Geometry: final body of the model. Coordinates: model frame, mm. Round coordinates to 2 decimals unless told otherwise and drop trailing zeros. Order: outer loops, then holes, each group sorted by start corner. A loop starts at its lowest first (then second) coordinate and runs counter-clockwise, first axis right, second up. Notation, with made-up numbers: (73.25, 42.25) - (129.25, 42.25) arc R28 ccw to (129.25, 77.25) - close; hole circle Ø10 at (3, 32). An arc over 180 degrees is marked (long way). Put each result on its own line as item: value. Start each with the question number.
(1) Section A-A (x = -83.5). Output: boundary loops of the cut face in (y, z) (3 decimals).
(2) Material intervals for L1, parallel to X at y = -2.5, z = -4.5; L2, parallel to Z at x = -83, y = -0.8, sorted ascending. Write a range as [from, to].
(3) Pin query (flat end, axial travel): P1, Ø1.5, axis at y = -2, z = -2.5, coming from the -X side; P2, Ø1.6, axis at x = 206.5, y = -1, coming from the -Z side; P3, Ø1, axis at y = -1.5, z = -39.5, coming from the +X side. Return the tip coordinate at first contact, or that it passes through.
from build123d import *

# Parameters (mm, degrees)
F1_DEPTH = 3.175


# Not quite as in the source:
# - ends of sketch curves that miss each other by under 0.0002 mm in the source are joined


with BuildPart() as f1:
    # F0 (on Front) → F1 (new body)
    with BuildSketch(Plane.XZ):
        Polygon((148.5900335276, 41.2750068545), (123.8250335276, 41.2750068545), (123.8250335276, 38.1000068545), (99.0600335276, 38.1000068545), (99.0600335276, 41.2750068545), (74.2950335276, 41.2750068545), (74.2950335276, 38.1000068545), (49.5300335276, 38.1000068545), (49.5300335276, 41.2750068545), (24.7650335276, 41.2750068545), (24.7650335276, 38.1000068545), (3.35276e-05, 38.1000068545), (3.35276e-05, 41.2750068545), (-24.7649664724, 41.2750068545), (-24.7649664724, 38.1000068545), (-49.5299664724, 38.1000068545), (-49.5299664724, 41.2750068545), (-74.2949664724, 41.2750068545), (-74.2949664724, 38.1000068545), (-99.0599664724, 38.1000068545), (-99.0599664724, 41.2750068545), (-123.8249664724, 41.2750068545), (-123.8249664724, 38.1000068545), (-148.5899664724, 38.1000068545), (-148.5899664724, 41.2750068545), (-173.3549664724, 41.2750068545), (-173.3549664724, 38.1000068545), (-198.1199664724, 38.1000068545), (-198.1199664724, 41.2750068545), (-222.8849664724, 41.2750068545), (-222.8849664724, 38.1000068545), (-247.6499664724, 38.1000068545), (-247.6499664724, 41.2750068545), (-272.4149664724, 41.2750068545), (-272.4149664724, 38.1000068545), (-297.1799664724, 38.1000068545), (-297.1799664724, 41.2750068545), (-321.9449664724, 41.2750068545), (-321.9449664724, 38.1000068545), (-346.7099664724, 38.1000068545), (-346.7099664724, 41.2750068545), (-371.4749664724, 41.2750068545), (-371.475, 38.1), (-371.475, 12.7), (-368.3, 12.7), (-368.3, -12.7), (-371.475, -12.7), (-371.475, -38.1), (-371.475031665, -41.2750032454), (-346.710031665, -41.2750032454), (-346.710031665, -38.1000032454), (-321.945031665, -38.1000032454), (-321.945031665, -41.2750032454), (-297.180031665, -41.2750032454), (-297.180031665, -38.1000032454), (-272.415031665, -38.1000032454), (-272.415031665, -41.2750032454), (-247.650031665, -41.2750032454), (-247.650031665, -38.1000032454), (-222.885031665, -38.1000032454), (-222.885031665, -41.2750032454), (-198.120031665, -41.2750032454), (-198.120031665, -38.1000032454), (-173.355031665, -38.1000032454), (-173.355031665, -41.2750032454), (-148.590031665, -41.2750032454), (-148.590031665, -38.1000032454), (-123.825031665, -38.1000032454), (-123.825031665, -41.2750032454), (-99.060031665, -41.2750032454), (-99.060031665, -38.1000032454), (-74.295031665, -38.1000032454), (-74.295031665, -41.2750032454), (-49.530031665, -41.2750032454), (-49.530031665, -38.1000032454), (-24.765031665, -38.1000032454), (-24.765031665, -41.2750032454), (-3.1665e-05, -41.2750032454), (-3.1665e-05, -38.1000032454), (24.764968335, -38.1000032454), (24.764968335, -41.2750032454), (49.529968335, -41.2750032454), (49.529968335, -38.1000032454), (74.294968335, -38.1000032454), (74.294968335, -41.2750032454), (92.075, -41.2750032454), (99.059968335, -41.2750032454), (99.059968335, -38.1000032454), (123.824968335, -38.1000032454), (123.824968335, -41.2750032454), (148.589968335, -41.2750032454), (148.589968335, -38.1000032454), (173.354968335, -38.1000032454), (173.354968335, -41.2750032454), (198.119968335, -41.2750032454), (198.119968335, -38.1000032454), (222.884968335, -38.1000032454), (222.884968335, -41.2750032454), (244.475, -41.2750032454), (247.649968335, -41.2750032454), (247.649968335, -38.1000032454), (272.414968335, -38.1000032454), (272.414968335, -41.2750032454), (297.179968335, -41.2750032454), (297.179968335, -38.1000032454), (321.944968335, -38.1000032454), (321.944968335, -41.2750032454), (346.709968335, -41.2750032453), (346.709968335, -38.1000032454), (371.474968335, -38.0999963909), (371.475, -12.7), (368.3, -12.7), (368.3, 12.7), (371.475, 12.7), (371.475, 38.1), (368.3, 38.1), (346.7100335276, 38.1), (346.7100335276, 41.2750068545), (321.9450335276, 41.2750068544), (321.9450335276, 38.1000068545), (297.1800335276, 38.1000068545), (297.1800335276, 41.2750068545), (272.4150335276, 41.2750068545), (272.4150335276, 38.1000068545), (247.6500335276, 38.1000068545), (247.6500335276, 41.2750068545), (222.8850335276, 41.2750068545), (222.8850335276, 38.1000068545), (198.1200335276, 38.1000068545), (198.1200335276, 41.2750068545), (173.3550335276, 41.2750068545), (173.3550335276, 38.1000068545), (148.5900335276, 38.1000068545), align=None)
    extrude(amount=F1_DEPTH)


solid = f1.part
Checks:
1. outline: (-3.175, -38.1) - (0, -38.1) - (0, 38.1) - (-3.175, 38.1) - close
2. L1: x = [-368.3, 368.3]
2. L2: z = [-38.1, 38.1]
3. P1: stops at x = -368.3
3. P2: stops at z = -38.1
3. P3: stops at x = 346.71
